Here's how the part is built. I have some questions about the finished solid (model axes, mm). A direction names the side the tool comes from. Round coordinates to 2 decimals unless told otherwise and drop trailing zeros. Write each loop counter-clockwise with the first axis right and the second up, starting at its lowest first coordinate (ties: lowest second). Pieces come first, ordered by that corner, then holes. Notation, with made-up numbers: (42.5, 43.25) -> (55.5, 43.25) arc R16 cw to (55.5, 48.25) -> close; hole circle Ø11 at (25, -14). An arc over 180 degrees is marked (long way). Answer as CSV lines item,"result".
```python
from build123d import *

# Parameters (mm, degrees)
F0_R     = 38.1
F0_R_2   = 5.5626
F0_R_3   = 17.5006
F1_DEPTH = 12.7
F0_R_4   = 3.3782
F2_DEPTH = 6.35
F0_R_5   = 9.525
F3_DEPTH = 1.8288
F4_SIZE  = 1.27


with BuildPart() as f1:
    # F0 (on Top) → F1 (new body)
    with BuildSketch(Plane.XY):
        Circle(F0_R)
        with Locations((-17.78, -23.241)):
            Circle(F0_R_2, mode=Mode.SUBTRACT)
        with Locations((17.78, -23.241)):
            Circle(F0_R_2, mode=Mode.SUBTRACT)
        with Locations((-17.78, 23.241)):
            Circle(F0_R_2, mode=Mode.SUBTRACT)
        Circle(F0_R_3, mode=Mode.SUBTRACT)
        with Locations((17.78, 23.241)):
            Circle(F0_R_2, mode=Mode.SUBTRACT)
    extrude(amount=F1_DEPTH)

    # F0 (on Top) → F2 (join)
    with BuildSketch(Plane.XY):
        with Locations((-17.78, 23.241)):
            Circle(F0_R_2)
        with Locations((-17.78, 23.241)):
            Circle(F0_R_4, mode=Mode.SUBTRACT)
        with Locations((17.78, 23.241)):
            Circle(F0_R_2)
        with Locations((17.78, 23.241)):
            Circle(F0_R_4, mode=Mode.SUBTRACT)
        with Locations((17.78, -23.241)):
            Circle(F0_R_2)
        with Locations((17.78, -23.241)):
            Circle(F0_R_4, mode=Mode.SUBTRACT)
        with Locations((-17.78, -23.241)):
            Circle(F0_R_2)
        with Locations((-17.78, -23.241)):
            Circle(F0_R_4, mode=Mode.SUBTRACT)
    extrude(amount=F2_DEPTH)

    # F0 (on Top) → F3 (join)
    with BuildSketch(Plane.XY):
        Circle(F0_R_3)
        Circle(F0_R_5, mode=Mode.SUBTRACT)
    extrude(amount=F3_DEPTH)

    # F4
    f4_edges = [f1.edges().sort_by_distance(p)[0] for p in [
        (-38.1, 0, 12.7),
        (-38.1, 0, 0),
    ]]
    chamfer(f4_edges, length=F4_SIZE)


solid = f1.part
```
1. If we mould it in two halves opening along X, with no side actions, what happens to faces 1 (the face through (8, -8, 0)), 2 (the face through (-18.99, -28.67, 9.48)), 3 (the face through (-14.558, -22.226, 3.131)), 4 (the face through (-30.235, -23.183, 6.279))? For each: released by +X, released by -X, zero draft, split by the parting line, or undercut.
Numbers:
face 1,"zero draft"
face 2,"undercut"
face 3,"undercut"
face 4,"split by the parting line"
2. Suppose I cut it at A-A on x = 0. Please give me the cut outline in (y, z) (3 decimals).
Numbers:
outline,"(-38.1, 1.27) -> (-36.83, 0) -> (-9.525, 0) -> (-9.525, 1.829) -> (-17.501, 1.829) -> (-17.501, 12.7) -> (-36.83, 12.7) -> (-38.1, 11.43) -> close; (9.525, 0) -> (36.83, 0) -> (38.1, 1.27) -> (38.1, 11.43) -> (36.83, 12.7) -> (17.501, 12.7) -> (17.501, 1.829) -> (9.525, 1.829) -> close"
3. Suppose I cut it at C-C on z = 8.25. Please give me the cut outline in (x, y).
Numbers:
outline,"circle Ø76.2 at (0, 0); hole circle Ø11.13 at (-17.78, -23.24); hole circle Ø11.13 at (-17.78, 23.24); hole circle Ø35 at (0, 0); hole circle Ø11.13 at (17.78, -23.24); hole circle Ø11.13 at (17.78, 23.24)"
4. On a 3-axis mill with a long thin cutter (end or side, diameter ignored), from which of +Z, -Z, +X, -X, +Y, -Y can I reach the whole of each face in a straight line? I mean faces 5 (the face through (14.405, 23.39, 3.131)), 6 (the face through (13.366, 19.856, 9.481)). Say none if no direction works.
Numbers:
face 5,"+Z, -Z"
face 6,"+Z"
5. If I drill on line 1 (X direction, y = 26, z = 4); line 2 (Y direction, x = -17.78, z = 9); line 3 (X direction, y = 0.5, z = 6.25), over which ranges is the centre line in solid material (lowest first)?
Numbers:
line 1,"x = -27.85 to -19.73, -15.83 to 15.83, 19.73 to 27.85"
line 2,"y = -33.7 to -28.8, -17.68 to 17.68, 28.8 to 33.7"
line 3,"x = -38.1 to -17.49, 17.49 to 38.1"
6. For pin 1 Ø22 at (x, y) = (0, 0) entering from +Z; pin 2 Ø5 at (x, z) = (-23, 11) entering from -Y; pin 3 Ø2 at (y, z) = (-2.5, 11) entering from +X; pin 4 Ø6 at (x, y) = (-17.78, 23.241) entering from -Z, each with a flat end and sliding along its axis, tell me the tip position at first contact or that it passes through.
Numbers:
pin 1,"stops at z = 1.83"
pin 2,"stops at y = -32.11"
pin 3,"stops at x = 38.07"
pin 4,"passes through"
